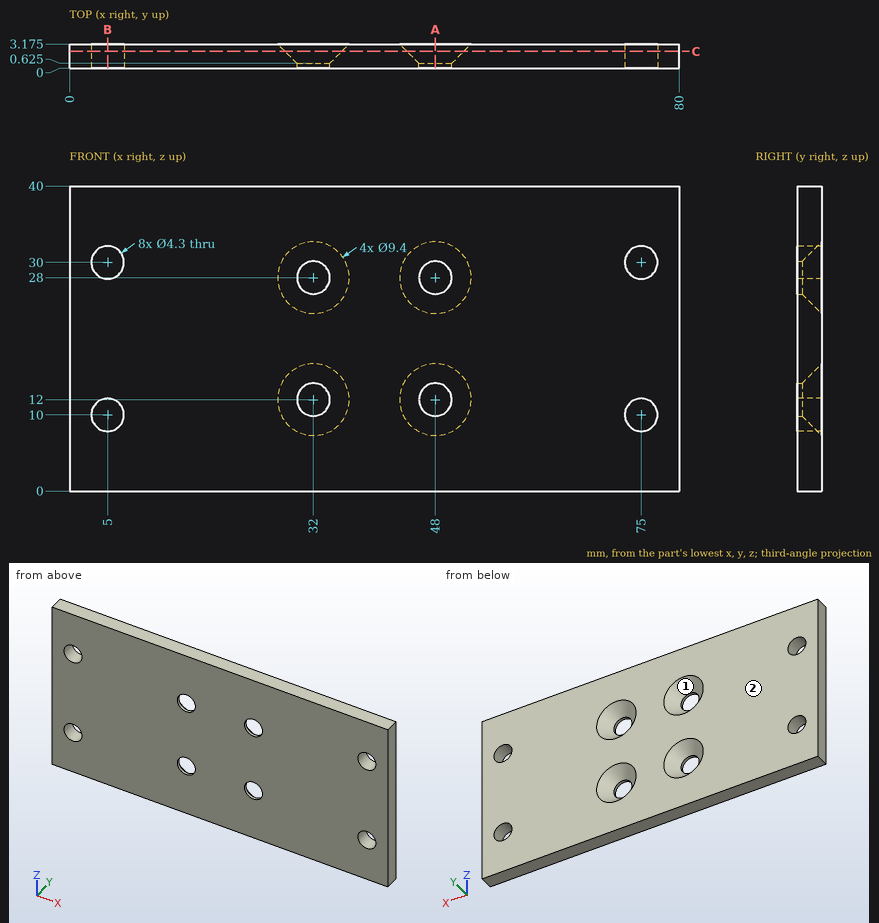
Input: dimensioned drawing with shaded views. Units: mm. Origin: part minimum x, y, z. Coordinates: 2 decimals unless noted, no trailing zeros. Loops run counter-clockwise (first coordinate to the right, second up) from the corner with the lowest first, then second, coordinate; pieces in that order, holes last.
Q1. Section A-A, the plane x = 48. Return the cut outline in (y, z) (3 decimals), and give its area (3 significant figures).
Results are:
outline: (0, 0) - (3.175, 0) - (3.175, 7.3) - (0.625, 9.85) - (0, 9.85) - close; (0, 14.15) - (0.625, 14.15) - (3.175, 16.7) - (3.175, 23.3) - (0.625, 25.85) - (0, 25.85) - close; (0, 30.15) - (0.625, 30.15) - (3.175, 32.7) - (3.175, 40) - (0, 40) - close
area: 86.7 mm2
Q2. Section B-B, the plane x = 5. Return the cut outline in (y, z) (3 decimals).
Results are:
outline: (0, 0) - (3.175, 0) - (3.175, 7.85) - (0, 7.85) - close; (0, 12.15) - (3.175, 12.15) - (3.175, 27.85) - (0, 27.85) - close; (0, 32.15) - (3.175, 32.15) - (3.175, 40) - (0, 40) - close
Q3. Mould query, pull axis X, two halves, no side actions, for the marked faces 1 and 2. Classes: +X half, -X half, draft (parallel to the pull), parting line (faces both ways), or undercut.
Results are:
face 1: undercut
face 2: draft
Q4. Contact query for a flat-ended pin moving along its axis: pin 1 (4 mm diameter, centred on x = 48, z = 12, fed in from +Y). Output: stop coordinate, or through.
Results are:
pin 1: passes through
Q5. Line query: line 1 along Z through (x, y) = (32, 0.45); line 2 along Z through (x, y) = (75, 1.95); line 3 along X through (y, z) = (2.5, 30). Output: solid intervals per line, ascending.
Results are:
line 1: z = 0 to 9.85, 14.15 to 25.85, 30.15 to 40
line 2: z = 0 to 7.85, 12.15 to 27.85, 32.15 to 40
line 3: x = 0 to 2.85, 7.15 to 28.51, 35.49 to 44.51, 51.49 to 72.85, 77.15 to 80
Q6. Section C-C, the plane y = 2.2. Give the number of separate pieces and of enclosed holes in the cut face, and give its area (3 significant figures).
Results are:
separate pieces: 1
enclosed holes: 8
area: 2,970 mm2
